Autodesk Inventor part; units mm, degrees
ref_plane "YZ Plane" through (0, 0, 0) normal (1, 0, 0) x (0, 1, 0)
ref_plane "XZ Plane" through (0, 0, 0) normal (0, 1, 0) x (-1, 0, 0)
ref_plane "XY Plane" through (0, 0, 0) normal (0, 0, 1) x (1, 0, 0)
ref_plane "Plano de trabalho1" through (0, 0, 0) normal (0, 0, 1) x (1, 0, 0)
sketch "Esboço1" plane through (0, 0, 0) normal (0, 0, 1) x (1, 0, 0)
  circle A0 centre (0, 9.5) radius 2.6
  line L0 (-7.5, -1.5) -> (-7.5, 1.5)
  line L1 (7.5, -1.5) -> (-7.5, -1.5)
  line L2 (7.5, 1.5) -> (7.5, -1.5)
  line L3 (-7.5, 1.5) -> (7.5, 1.5)
  circle A1 centre (0, -9.5) radius 2.6
  line L4 (-7.5, 1.5) -> (7.5, 1.5)
  line L5 (7.5, 1.5) -> (7.5, 15.5)
  line L6 (-7.5, 15.5) -> (-7.5, 1.5)
  circle A2 centre (0, 9.5) radius 2.1
  line L7 (7.5, -1.5) -> (-7.5, -1.5)
  line L8 (-7.5, -1.5) -> (-7.5, -15.5)
  line L9 (7.5, -15.5) -> (7.5, -1.5)
  circle A3 centre (0, -9.5) radius 2.1
  line L10 (-7.5, 15.5) -> (7.5, 15.5)
  line L11 (7.5, 15.5) -> (7.5, -15.5)
  line L12 (7.5, -15.5) -> (-7.5, -15.5)
  line L13 (-7.5, -15.5) -> (-7.5, 15.5)
  point P0 (0, 0)
  dimension "d0" = 14
  dimension "d1" = 14
  dimension "d7" = 5.2
  dimension "d8" = 5.2
extrude "Extrusão1" add sketch "Esboço1" along normal blind 4 contours L0 L3 L2 L1 | L1 L9 L12 L8 | L6 L10 L5 L3
extrude "Extrusão2" cut sketch "Esboço1" along normal blind 1.5 contours L0 L3 L2 L1
fillet "Arredondamento1" radius 2 4 edges at (-7.5, 15.5, 2) (7.5, 15.5, 2) (-7.5, -15.5, 2) (7.5, -15.5, 2)
fillet "Arredondamento2" radius 1.5 2 edges at (0, -1.5, 1.5) (0, 1.5, 1.5)
equation "\"d1\" = d0"
equation "\"d8\" = d7"
properties part number "tampa_suporte_termopar"
Geometry: final body of the model. Coordinates: model frame, mm. A direction names the side the tool comes from. Give positions to 0.01 mm unless a question says otherwise; leave off trailing zeros. Write each loop counter-clockwise with the first axis right and the second up, starting at its lowest first coordinate (ties: lowest second). Pieces come first, ordered by that corner, then holes. Notation, with made-up numbers: (19.5, -7) - (69.5, -7) arc R26 cw to (69.5, 32) - close; hole circle Ø8 at (-11, 39.5). An arc over 180 degrees is marked (long way). Return JSON: item names as keys, results as strings. Group by question number.
1) Section A-A on z = 1.1. Return the cut outline in (x, y), plus the area to 3 significant figures.
2) Section B-B on y = 9.5. Return the cut outline in (x, z).
3) Mould query, pull axis Y, two halves, no side actions, for faces 1 (the cylindrical face through (-0.11, -1.07, 1.05)), 2 (the cylindrical face through (6.93, 14.9, 2.03)), 3 (the cylindrical face through (6.9, -14.93, 2.03)), 4 (the flat face through (-7.5, 0, 2)). Classes: released by +Y, released by -Y, zero draft, split by the parting line, or undercut.
4) Section C-C on x = 0. State how many separate pieces and enclosed holes the cut face has, plus the area to 3 significant figures.
5) Line query: line 1 (Y direction, x = 0, z = 2.8); line 2 (Y direction, x = -0.5, z = 0.9); line 3 (Y direction, x = 2, z = 0.5). Output: solid intervals per line, ascending.
6) Set-up query: faces 5 (the cylindrical face through (0.11, 1.07, 1.05)), 6 (the cylindrical face through (-0.56, 12.04, 1.97)). Return all of +Z, -Z, +X, -X, +Y, -Y with unobstructed straight access to the full face (end or side cutting, diameter ignored); none if empty.
Filled in:
{
 "1": {"outline": "(-7.5, -13.5) arc R2 ccw to (-5.5, -15.5) - (5.5, -15.5) arc R2 ccw to (7.5, -13.5) - (7.5, -1.02) - (-7.5, -1.02) - close; (-7.5, 1.02) - (7.5, 1.02) - (7.5, 13.5) arc R2 ccw to (5.5, 15.5) - (-5.5, 15.5) arc R2 ccw to (-7.5, 13.5) - close; hole circle Ø5.2 at (0, -9.5); hole circle Ø5.2 at (0, 9.5)", "area": "388 mm^2"},
 "2": {"outline": "(-7.5, 0) - (-2.6, 0) - (-2.6, 4) - (-7.5, 4) - close; (2.6, 0) - (7.5, 0) - (7.5, 4) - (2.6, 4) - close"},
 "3": {"face 1": "undercut", "face 2": "released by +Y", "face 3": "released by -Y", "face 4": "zero draft"},
 "4": {"separate pieces": "3", "enclosed holes": "0", "area": "78.9 mm^2"},
 "5": {"line 1": "y = -15.5 to -12.1, -6.9 to 6.9, 12.1 to 15.5", "line 2": "y = -15.5 to -12.05, -6.95 to -1.2, 1.2 to 6.95, 12.05 to 15.5", "line 3": "y = -15.5 to -11.16, -7.84 to -1.41, 1.41 to 7.84, 11.16 to 15.5"},
 "6": {"face 5": "-Z, +X, -X", "face 6": "+Z, -Z"}
}
